Verification items for the finished model (mm, model axes). Face numbers are marked on the shaded views. A direction names the side the tool comes from. Round coordinates to 2 decimals unless told otherwise and drop trailing zeros. Order: outer loops, then holes, each group sorted by start corner. A loop starts at its lowest first (then second) coordinate and runs counter-clockwise, first axis right, second up. Notation, with made-up numbers: (-30, 63) -> (0, 63) arc R26 cw to (0, 86) -> close; hole circle Ø7 at (32.25, 57). An arc over 180 degrees is marked (long way). Put each result on its own line as item: value.
from build123d import *

# Parameters (mm, degrees)
F0_R      = 1.657861898
F0_R_2    = 1.5637435582
F0_R_3    = 1.5
F0_R_4    = 1.6928931088
F1_DEPTH  = 2
F2_W      = 12
F2_H      = 12
F3_DEPTH  = 8
F4_R      = 3.1469960725
F5_DEPTH  = 10
F6_W      = 8.1816576421
F6_H      = 15.9170441329
F6_W_2    = 6.694085896
F6_H_2    = 15.9170404077
F6_W_3    = 9.9330767989
F6_H_3    = 9.9667422473
F6_W_4    = 9.3853771687
F6_H_4    = 10.1155005395
F7_DEPTH  = 10
F8_R      = 6.2283008091
F8_R_2    = 6.1225151743
F9_DEPTH  = 15
F10_R     = 4.0154432522
F10_R_2   = 3.7333835988
F11_DEPTH = 10


with BuildPart() as f1:
    # F0 (on Top) → F1 (new body)
    with BuildSketch(Plane.XY):
        Polygon((-70.0199790299, 79.3929218054), (-70.0199790299, 26.3929218054), (32.9800209701, 26.3929218054), (32.9800209701, 79.3929218054), (17.9800209701, 79.3929218054), align=None)
        with Locations((-67.0199790299, 29.3929218054)):
            Circle(F0_R, mode=Mode.SUBTRACT)
        with Locations((29.9800209701, 29.3929218054)):
            Circle(F0_R_2, mode=Mode.SUBTRACT)
        with Locations((-67.0199790299, 76.3929218054)):
            Circle(F0_R_3, mode=Mode.SUBTRACT)
        with Locations((29.9800209701, 76.3929218054)):
            Circle(F0_R_4, mode=Mode.SUBTRACT)
    extrude(amount=F1_DEPTH)

    # F2 (on face) → F3 (join)
    with BuildSketch(Plane(origin=(0, 79.3929218054, 0), x_dir=(-1, 0, 0), z_dir=(0, 1, 0))):
        with Locations((54.0199790299, 8)):
            Rectangle(F2_W, F2_H)
        with Locations((30.0199790299, 8)):
            Rectangle(F2_W, F2_H)
        with Locations((6.0199790299, 8)):
            Rectangle(F2_W, F2_H)
        with Locations((-17.9800209701, 8)):
            Rectangle(F2_W, F2_H)
    extrude(amount=-F3_DEPTH)

    # F4 (on face) → F5 (join)
    with BuildSketch(Plane(origin=(0, 79.3929218054, 0), x_dir=(-1, 0, 0), z_dir=(0, 1, 0))):
        with Locations((-17.9800209701, 7.9124979675)):
            Circle(F4_R)
        with Locations((6.0199790299, 7.9124979675)):
            Circle(F4_R)
        with Locations((30.0199790299, 7.9124979675)):
            Circle(F4_R)
        with Locations((54.0199790299, 7.9124979675)):
            Circle(F4_R)
    extrude(amount=F5_DEPTH)

    # F6 (on face) → F7 (join)
    with BuildSketch(Plane.XY.offset(2)):
        with Locations((-63.6116955429, 63.0893874913)):
            Rectangle(F6_W, F6_H)
        with Locations((-64.0579722822, 42.412109673)):
            Rectangle(F6_W_2, F6_H_2)
        with Locations((28.7498049438, 56.0977887362)):
            Rectangle(F6_W_3, F6_H_3)
        with Locations((29.0709845722, 43.2302746922)):
            Rectangle(F6_W_4, F6_H_4)
    extrude(amount=F7_DEPTH)

    # F8 (on face) → F9 (join)
    with BuildSketch(Plane.XY.offset(2)):
        with Locations((-44.3476177752, 48.1392666698)):
            Circle(F8_R)
        with Locations((-43.4550717473, 34.304831177)):
            Circle(F8_R_2)
    extrude(amount=F9_DEPTH)

    # F10 (on face) → F11 (join)
    with BuildSketch(Plane.YZ.offset(33.7163433433)):
        with Locations((56.0977887362, 7)):
            Circle(F10_R)
        with Locations((43.5904636979, 7.3108654469)):
            Circle(F10_R_2)
    extrude(amount=F11_DEPTH)


solid = f1.part
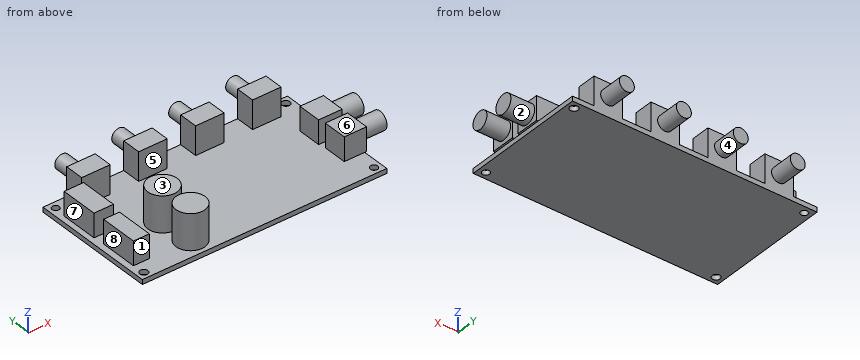
Item 1: Tool access check on the marked faces 4, 5, 6, 7 and 8. Record the directions out of +Z, -Z, +X, -X, +Y, -Y that give a thin tool (end or side, any length) a straight path to the whole face; none if there is none.
Check sheet entries:
face 4: +Y
face 5: +Z, +X, -X, -Y
face 6: +Z, +X, +Y, -Y
face 7: +Z, -X, +Y, -Y
face 8: +Z, -X, -Y
Item 2: Section check C-C on z = 15.5. Record the boundary of the cut face in (x, y).
Check sheet entries:
outline: circle Ø12.46 at (-44.35, 48.14); circle Ø12.25 at (-43.46, 34.3)
Item 3: Release check for a two-part mould opening along Y. For the marked faces 1, 2 and 3 record: +Y half, -Y half, draft (parallel to the pull), parting line (faces both ways), or undercut.
Check sheet entries:
face 1: -Y half
face 2: undercut
face 3: draft
Item 4: Material ranges on L1, parallel to X at y = 74.5, z = 13.75; L2, parallel to X at y = 47.5, z = 9; L3, parallel to Z at x = 13, y = 42.5, recorded low to high. Write a range as [from, to].
Check sheet entries:
L1: x = [-60.02, -48.02], [-36.02, -24.02], [-12.02, -0.02], [11.98, 23.98]
L2: x = [-67.41, -60.71], [-50.54, -38.15], [24.38, 33.76]
L3: z = [0, 2]
Item 5: Section check B-B on y = 68. Record the boundary of the cut face in (x, z), then the cut area to 3 significant figures.
Check sheet entries:
outline: (-70.02, 0) -> (32.98, 0) -> (32.98, 2) -> (-59.52, 2) -> (-59.52, 12) -> (-67.7, 12) -> (-67.7, 2) -> (-70.02, 2) -> close
area: 288 mm^2
Item 6: Section check A-A on x = 26. Record the boundary of the cut face in (y, z).
Check sheet entries:
outline: (26.39, 0) -> (79.39, 0) -> (79.39, 2) -> (61.08, 2) -> (61.08, 12) -> (51.11, 12) -> (51.11, 2) -> (48.29, 2) -> (48.29, 12) -> (38.17, 12) -> (38.17, 2) -> (26.39, 2) -> close
Item 7: Section check D-D on z = 9. State how many separate pieces and enclosed holes the cut face has, then the cut area to 3 significant figures.
Check sheet entries:
separate pieces: 10
enclosed holes: 0
area: 1,430 mm^2
Item 8: Gauge pin test, flat ends, axial feed: pin 1 Ø2.5 at (x, y) = (29.98, 76.39) entering from -Z; pin 2 Ø6.5 at (x, y) = (17, 73.5) entering from +Z; pin 3 Ø2 at (x, y) = (5, 79.5) entering from +Z; pin 4 Ø3 at (x, y) = (29, 41) entering from +Z. Record the tip position at first contact, or that the pin passes through.
Check sheet entries:
pin 1: passes through
pin 2: stops at z = 14
pin 3: stops at z = 2
pin 4: stops at z = 12
